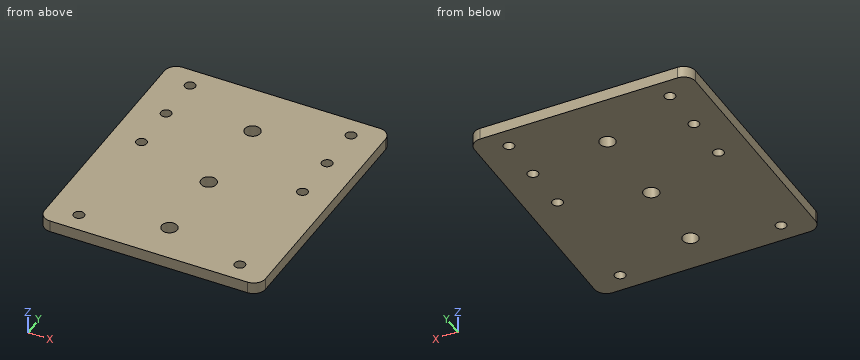
from build123d import *

# Parameters (mm, degrees)
BOSS_EXTRU_1_DEPTH = 5
D_GAGEMENT_M61_D   = 6.6
D_GAGEMENT_M41_D   = 4.5


with BuildPart() as part:
    # Esquisse1 → Boss.-Extru.1 (new body)
    with BuildSketch(Plane.XY):
        with BuildLine():
            Line((-42, 54.5), (42, 54.5))
            ThreePointArc((42, 54.5), (45.535533906, 53.035533906), (47, 49.5))
            Line((47, 49.5), (47, -49.5))
            ThreePointArc((47, -49.5), (45.535533906, -53.035533906), (42, -54.5))
            Line((42, -54.5), (-42, -54.5))
            ThreePointArc((-42, -54.5), (-45.535533906, -53.035533906), (-47, -49.5))
            Line((-47, -49.5), (-47, 49.5))
            ThreePointArc((-47, 49.5), (-45.535533906, 53.035533906), (-42, 54.5))
        make_face()
    extrude(amount=BOSS_EXTRU_1_DEPTH)

    # Dégagement M61 (through all)
    with Locations(Plane.XY.offset(5)):
        with Locations((0, 30.929411148), (0, -37.544992042), (0, -5.15832988)):
            Hole(D_GAGEMENT_M61_D / 2)

    # Dégagement M41 (through all)
    with Locations(Plane.XY.offset(5)):
        with Locations((34.336239969, 45.611301296), (34.336239969, 25.844548243), (34.336239969, 5.572681811), (34.336239969, -46.046219335), (-34.125150255, -46.046219335), (-34.125150255, 5.572681811), (-34.125150255, 25.844548243), (-34.125150255, 45.611301296)):
            Hole(D_GAGEMENT_M41_D / 2)


solid = part.part
Source: CAD feature listing. Evaluate the final solid. Frame: model axes, mm. Give positions to 0.01 mm unless a question says otherwise; leave off trailing zeros. Write each loop counter-clockwise with the first axis right and the second up, starting at its lowest first coordinate (ties: lowest second). Pieces come first, ordered by that corner, then holes. Notation, with made-up numbers: (-24, -18.75) -> (20, -18.75) arc R16 ccw to (20, -4.75) -> close; hole circle Ø2 at (72, 38). An arc over 180 degrees is marked (long way). Write item = value, one per line.
Q1. Cut plane A-A on x = 0. Return loops of the section in (y, z) (3 decimals).
Here are the results:
outline = (-54.5, 0) -> (-40.845, 0) -> (-40.845, 5) -> (-54.5, 5) -> close; (-34.245, 0) -> (-8.458, 0) -> (-8.458, 5) -> (-34.245, 5) -> close; (-1.858, 0) -> (27.629, 0) -> (27.629, 5) -> (-1.858, 5) -> close; (34.229, 0) -> (54.5, 0) -> (54.5, 5) -> (34.229, 5) -> close
Q2. Cut plane C-C on x = -33.5. Return loops of the section in (y, z).
Here are the results:
outline = (-54.5, 0) -> (-48.21, 0) -> (-48.21, 5) -> (-54.5, 5) -> close; (-43.88, 0) -> (3.41, 0) -> (3.41, 5) -> (-43.88, 5) -> close; (7.73, 0) -> (23.68, 0) -> (23.68, 5) -> (7.73, 5) -> close; (28.01, 0) -> (43.45, 0) -> (43.45, 5) -> (28.01, 5) -> close; (47.77, 0) -> (54.5, 0) -> (54.5, 5) -> (47.77, 5) -> close
Q3. Cut plane B-B on z = 2.35. State how many separate pieces and enclosed holes the cut face has, then the cut area to 3 significant figures.
Here are the results:
separate_pieces = 1
enclosed_holes = 11
area = 9,990 mm²
Q4. Line query: line 1 (X direction, y = 45.5, z = 2.05); line 2 (X direction, y = 24.5, z = 3.15); line 3 (Y direction, x = -42.5, z = 2.2). Output: solid intervals per line, ascending. Write a range as from..to.
Here are the results:
line_1 = -47..-36.37, -31.88..32.09, 36.58..47
line_2 = -47..-35.93, -32.32..32.53, 36.14..47
line_3 = -54.47..54.47
